Work out the finished part from the listing and answer in its coordinate system (mm). Face numbers are marked on the shaded views. A direction names the side the tool comes from. Round coordinates to 2 decimals unless told otherwise and drop trailing zeros. Write each loop counter-clockwise with the first axis right and the second up, starting at its lowest first coordinate (ties: lowest second). Pieces come first, ordered by that corner, then holes. Notation, with made-up numbers: (-3.75, 82.5) -> (12.25, 82.5) arc R22 cw to (12.25, 114.5) -> close; hole circle Ø10 at (1, 83.5). An arc over 180 degrees is marked (long way). One line per question, with ' | ' between items. Start each with the question number.
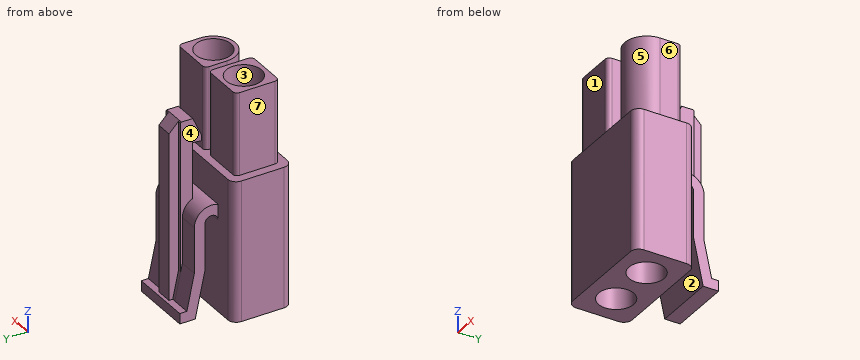
```python
from build123d import *

# Parameters (mm, degrees)
SKETCH1_W               = 13.32
SKETCH1_H               = 7.14
BOSS_EXTRUDE1_DEPTH     = 16.89
SKETCH2_W               = 5.27
SKETCH2_H               = 5.27
BOSS_EXTRUDE2_DEPTH     = 9.94
CUT_EXTRUDE1_DEPTH      = 19.503313217
CUT_EXTRUDE1_DEPTH_BACK = 19.503313217
SKETCH3_R               = 2.12
BOSS_EXTRUDE3_DEPTH     = 3.77
BOSS_EXTRUDE4_DEPTH     = 1.415
CUT_EXTRUDE3_DEPTH      = 0.415
CUT_EXTRUDE4_DEPTH      = 0.415
FILLET1_R               = 1
FILLET2_R               = 0.5


with BuildPart() as part:
    # Sketch1 → Boss-Extrude1 (new body)
    with BuildSketch(Plane.XY):
        Rectangle(SKETCH1_W, SKETCH1_H)
    extrude(amount=-BOSS_EXTRUDE1_DEPTH)

    # Sketch2 → Boss-Extrude2 (add)
    with BuildSketch(Plane.XY):
        with BuildLine():
            Line((0.35, 2.635), (0.35, 0))
            ThreePointArc((0.35, 0), (2.985, -2.635), (5.62, 0))
            Line((5.62, 0), (5.62, 2.635))
            Line((5.62, 2.635), (0.35, 2.635))
        make_face()
        with Locations((-2.985, 0)):
            Rectangle(SKETCH2_W, SKETCH2_H)
    extrude(amount=BOSS_EXTRUDE2_DEPTH)

    # Sketch3 → Cut-Extrude1 (cut, two sides: drawn at the far end of the back side and taken through both)
    with BuildSketch(Plane.XY.offset(-CUT_EXTRUDE1_DEPTH_BACK)):
        with Locations((2.985, 0)):
            Circle(SKETCH3_R)
        with Locations((-2.985, 0)):
            Circle(SKETCH3_R)
    extrude(amount=CUT_EXTRUDE1_DEPTH + CUT_EXTRUDE1_DEPTH_BACK, mode=Mode.SUBTRACT)

    # Sketch4 → Boss-Extrude3 (add, symmetric)
    with BuildSketch(Plane(origin=(0, 0, 0), x_dir=(0, 0, -1), z_dir=(1, 0, 0))):
        with BuildLine():
            Line((5.885, 5.18), (11.5212493, 5.18))
            Line((11.5212493, 5.18), (16.89, 6.32))
            Line((16.89, 6.32), (16.89, 8.18))
            Line((16.89, 8.18), (15.64, 8.18))
            Line((15.64, 8.18), (15.64, 7.332444585))
            Line((15.64, 7.332444585), (11.39, 6.43))
            Line((11.39, 6.43), (5.885, 6.43))
            ThreePointArc((5.885, 6.43), (4.170750893, 5.508302696), (3.99423296, 3.57))
            Line((3.99423296, 3.57), (5.885, 3.57))
            ThreePointArc((5.885, 3.57), (5.08, 4.375), (5.885, 5.18))
        make_face()
    extrude(amount=BOSS_EXTRUDE3_DEPTH, both=True)

    # Sketch5 → Boss-Extrude4 (add, symmetric)
    with BuildSketch(Plane(origin=(0, 0, 0), x_dir=(0, 0, -1), z_dir=(1, 0, 0))):
        Polygon((15.64, 7.78), (-4.372563133, 7.78), (-5.61, 6.542563133), (-5.61, 5.18), (-3.36, 4.15), (-2.61, 4.15), (-2.71, 5.18), (5.503211952, 5.18), (15.64, 7.332444585), align=None)
    extrude(amount=BOSS_EXTRUDE4_DEPTH, both=True)

    # Sketch7 → Cut-Extrude3 (cut)
    with BuildSketch(Plane.ZY.offset(1.415)):
        Polygon((4.372563133, 7.78), (5.522563133, 6.63), (-12.331886088, 6.63), (-15.64, 7.332444585), (-15.64, 7.78), align=None)
    extrude(amount=-CUT_EXTRUDE3_DEPTH, mode=Mode.SUBTRACT)

    # Sketch8 → Cut-Extrude4 (cut)
    with BuildSketch(Plane(origin=(1.415, 0, 0), x_dir=(0, 0, -1), z_dir=(1, 0, 0))):
        Polygon((-4.372563133, 7.78), (-5.522563133, 6.63), (12.331886088, 6.63), (15.64, 7.332444585), (15.64, 7.78), align=None)
    extrude(amount=-CUT_EXTRUDE4_DEPTH, mode=Mode.SUBTRACT)

    # Fillet1
    fillet1_edges = [part.edges().sort_by_distance(p)[0] for p in [
        (-6.66, -3.57, -8.445),
        (6.66, -3.57, -8.445),
        (6.66, 3.57, -8.445),
        (-6.66, 3.57, -8.445),
    ]]
    fillet(fillet1_edges, radius=FILLET1_R)

    # Fillet2
    fillet2_edges = [part.edges().sort_by_distance(p)[0] for p in [
        (-5.62, -2.635, 4.97),
        (-0.35, -2.635, 4.97),
        (-0.35, 2.635, 4.97),
        (-5.62, 2.635, 4.97),
        (5.62, 2.635, 4.97),
        (0.35, 2.635, 4.97),
    ]]
    fillet(fillet2_edges, radius=FILLET2_R)


solid = part.part
```
(1) A cutting plane is placed at A-A, the plane z = -9. Determine the outline of the cut face in (x, y) (3 decimals), then the cut area to 3 significant figures.
(2) A cutting plane is placed at D-D, the plane y = -1. Determine the outline of the cut face in (x, z), then the cut area to 3 significant figures.
(3) A cutting plane is placed at B-B, the plane y = 1. Determine the outline of the cut face in (x, z), then the cut area to 3 significant figures.
(4) Consider L1, parallel to X at y = 0, z = -5.5 (3 decimals); L2, parallel to Y at x = 1.25, z = -6.75; L3, parallel to Y at x = 1.75, z = -10.25. Determine where each line is inside the solid, lowest interval first.
(5) Given pin 1 Ø5 at (y, z) = (5, -10.5) entering from +X; pin 2 Ø1.2 at (y, z) = (5, 1) entering from -X (3 decimals); pin 3 Ø1 at (x, z) = (0, -6) entering from +Y; pin 4 Ø2.5 at (y, z) = (5, -5.5) entering from +X, each flat-ended and moving along its own axis, determine where each tip first touches the part or whether it passes through.
(6) A cutting plane is placed at C-C, the plane y = 7. Determine the outline of the cut face in (x, z) (3 decimals).
(7) The mould has two halves that part along Y. Classify the marked faces 1, 2, 3 and 4: +Y half, -Y half, draft (parallel to the pull), parting line (faces both ways), or undercut.
(8) For the marked faces 5, 6 and 7, determine the directions among +Z, -Z, +X, -X, +Y, -Y from which every point of the face is accessible in a straight line to the end or side of a thin tool.
Returned:
1) outline: (-6.66, -2.57) arc R1 ccw to (-5.66, -3.57) -> (5.66, -3.57) arc R1 ccw to (6.66, -2.57) -> (6.66, 2.57) arc R1 ccw to (5.66, 3.57) -> (-5.66, 3.57) arc R1 ccw to (-6.66, 2.57) -> close; (-3.77, 5.18) -> (3.77, 5.18) -> (3.77, 6.43) -> (1.415, 6.43) -> (1.415, 6.63) -> (1, 6.63) -> (1, 7.78) -> (-1, 7.78) -> (-1, 6.63) -> (-1.415, 6.63) -> (-1.415, 6.43) -> (-3.77, 6.43) -> close; hole circle Ø4.24 at (-2.985, 0); hole circle Ø4.24 at (2.985, 0) | area: 78.3 mm2
2) outline: (-6.66, -16.89) -> (-4.85, -16.89) -> (-4.85, 9.94) -> (-5.62, 9.94) -> (-5.62, 0) -> (-6.66, 0) -> close; (-1.12, -16.89) -> (1.12, -16.89) -> (1.12, 9.94) -> (0.55, 9.94) -> (0.55, 0) -> (-0.35, 0) -> (-0.35, 9.94) -> (-1.12, 9.94) -> close; (4.85, -16.89) -> (6.66, -16.89) -> (6.66, 0) -> (5.42, 0) -> (5.42, 9.94) -> (4.85, 9.94) -> close | area: 125 mm2
3) outline: (-6.66, -16.89) -> (-4.85, -16.89) -> (-4.85, 9.94) -> (-5.62, 9.94) -> (-5.62, 0) -> (-6.66, 0) -> close; (-1.12, -16.89) -> (1.12, -16.89) -> (1.12, 9.94) -> (0.35, 9.94) -> (0.35, 0) -> (-0.35, 0) -> (-0.35, 9.94) -> (-1.12, 9.94) -> close; (4.85, -16.89) -> (6.66, -16.89) -> (6.66, 0) -> (5.62, 0) -> (5.62, 9.94) -> (4.85, 9.94) -> close | area: 129 mm2
4) L1: -6.66 to -5.105, -0.865 to 0.865, 5.105 to 6.66 | L2: -3.57 to -1.22, 1.22 to 3.57, 5.18 to 6.63 | L3: -3.57 to -1.72, 1.72 to 3.57, 5.18 to 6.43
5) pin 1: x = 6.66 | pin 2: x = -1.415 | pin 3: y = 7.78 | pin 4: x = 3.77
6) outline: (-3.77, -16.89) -> (3.77, -16.89) -> (3.77, -14.074) -> (1, -14.074) -> (1, 5.153) -> (-1, 5.153) -> (-1, -14.074) -> (-3.77, -14.074) -> close
7) face 1: -Y half | face 2: undercut | face 3: undercut | face 4: draft
8) face 5: +Z, -Y | face 6: +Z, +X, +Y, -Y | face 7: +Z, -X, +Y, -Y
